Part model, mm, in its own coordinate system. A direction names the side the tool comes from. Coordinates: 2 decimals unless noted, no trailing zeros. Write each loop counter-clockwise with the first axis right and the second up, starting at its lowest first coordinate (ties: lowest second). Pieces come first, ordered by that corner, then holes. Notation, with made-up numbers: (39.25, -18.75) -> (48.25, -18.75) arc R20 cw to (48.25, -10.75) -> close; hole circle Ø7 at (44, 21). An arc over 180 degrees is marked (long way). Write item = value, one per line. Start each with the question number.
Q1. Pull direction Z, two halves, no side cores. Call faces 4 (the cylindrical face through (-31.2, 8.5, -0.1)), 5 (the flat face through (0, 3, 12.5)), 6 (the cylindrical face through (31.2, 8.7, 11.5)): released by +Z, released by -Z, zero draft, split by the parting line, or undercut.
Q2. Band-saw the part on B-B, the plane z = -0.5. List the corners of the cut face in (x, y).
Q3. Tool access for faces 1 (the cylindrical face through (31.3, 8.5, -0.1)), 2 (the flat face through (0, 3, -12.5)), 3 (the flat face through (0, 2, 10)): list every direction of +Z, -Z, +X, -X, +Y, -Y with a clear straight run to the whole face (end or side of a thin tool).
Q4. Band-saw the part on A-A, the plane x = 16.5. List the corners of the cut face in (y, z), plus the area to 3 significant figures.
Q5. Probe line 1 (Z direction, x = -24.5, y = 2.75); line 2 (X direction, y = 1.75, z = -1); line 3 (X direction, y = 5.5, z = 10.75). List the from-to ranges inside material, lowest first.
Q6. Band-saw the part on D-D, the plane y = 3. List the corners of the cut face in (x, z).
Q7. Band-saw the part on C-C, the plane y = 7. List the corners of the cut face in (x, z), plus the area to 3 significant figures.
Q8. Pin check, flat tip, straight feed: P1, Ø1.5, axis at x = 21, z = -3.5, coming from the +Y side. Stop position of the tip, or through.
Autodesk Inventor part; units mm, degrees
ref_plane "YZ Plane" through (0, 0, 0) normal (1, 0, 0) x (0, 1, 0)
ref_plane "XZ Plane" through (0, 0, 0) normal (0, 1, 0) x (-1, 0, 0)
ref_plane "XY Plane" through (0, 0, 0) normal (0, 0, 1) x (1, 0, 0)
sketch "Sketch1" plane through (0, 0, 0) normal (0, 1, 0) x (-1, 0, 0)
  line L0 (-35, -12.5) -> (35, -12.5)
  line L1 (35, -12.5) -> (35, 12.5)
  line L2 (35, 12.5) -> (-35, 12.5)
  line L3 (-35, 12.5) -> (-35, -12.5)
  line L4 (-35, -12.5) -> (35, 12.5) construction
  line L5 (35, -12.5) -> (-35, 12.5) construction
  line L6 (-24.5, -5) -> (24.5, -5) construction
  line L7 (24.5, -5) -> (24.5, 5) construction
  line L8 (24.5, 5) -> (-24.5, 5) construction
  line L9 (-24.5, 5) -> (-24.5, -5) construction
  line L10 (-24.5, -5) -> (24.5, 5) construction
  line L11 (24.5, -5) -> (-24.5, 5) construction
  circle A0 centre (24.5, 5) radius 2.25
  circle A1 centre (24.5, -5) radius 2.25
  circle A2 centre (-24.5, -5) radius 2.25
  circle A3 centre (-24.5, 5) radius 2.25
  line L12 (-20, -10) -> (20, -10)
  line L13 (20, -10) -> (20, 10)
  line L14 (20, 10) -> (-20, 10)
  line L15 (-20, 10) -> (-20, -10)
  line L16 (-20, -10) -> (20, 10) construction
  line L17 (20, -10) -> (-20, 10) construction
  point P0 (0, 0)
  dimension "d0" = 10
  dimension "d1" = 49
  dimension "d2" = 4.5
  dimension "d5" = 25
  dimension "d6" = 70
  dimension "d7" = 20
  dimension "d8" = 40
extrude "Extrusion1" add sketch "Sketch1" along normal blind 5
sketch "Sketch2" plane through (35, 0, -12.5) normal (0, 0, -1) x (-1, 0, 0)
  line L0 (62.5, 5) -> (62.5, 11)
  line L1 (62.5, 11) -> (70, 11)
  line L2 (70, 11) -> (70, 5)
  line L3 (70, 5) -> (62.5, 5)
  line L4 (35, -3.7897) -> (35, 10.3895) construction
  circle A0 centre (66.25, 11) radius 2.5
  line L5 (0, 5) -> (7.5, 5)
  circle A1 centre (66.25, 11) radius 2.3
  line L6 (7.5, 5) -> (7.5, 11)
  line L7 (7.5, 11) -> (0, 11)
  line L8 (0, 11) -> (0, 5)
  line L9 (0, 5) -> (7.5, 5)
  circle A2 centre (3.75, 11) radius 2.5
  circle A3 centre (3.75, 11) radius 2.3
  line L10 (0, 0) -> (70, 0)
  point P0 (35, 0)
  point P1 (35, 0)
  point P2 (68.75, 11)
  point P3 (63.75, 11)
  point P4 (35, 0)
  point P5 (6.05, 11)
  point P6 (1.45, 11)
  point P7 (1.25, 11)
  point P8 (6.25, 11)
  point P9 (68.55, 11)
  point P10 (63.95, 11)
  dimension "d9" = 5
  dimension "d10" = 7.5
  dimension "d12" = 6
  dimension "d18" = 0.2
extrude "Extrusion2" add sketch "Sketch2" against normal up to surface (25 mm away) contours L0 L1 A0 L2 L3 | L8 L7 A2 L6 L5
extrude "Extrusion4" add sketch "Sketch2" against normal blind 2 contours L1 A1 A0 | L7 A3 A2 picked at (64.2095, 9.7038) picked at (6.1368, 10.6171)
mirror "Mirror1" about plane through (0, 0, 0) normal (0, 0, 1) of "Extrusion4"
properties part number "Servo mount"
Ans:
q1.face_4 = undercut
q1.face_5 = released by +Z
q1.face_6 = zero draft
q2.outline = (-35, 0) -> (-20, 0) -> (-20, 5) -> (-27.5, 5) -> (-27.5, 11) -> (-28.75, 11) arc R2.5 cw to (-33.75, 11) -> (-35, 11) -> close; (20, 0) -> (35, 0) -> (35, 11) -> (33.75, 11) arc R2.5 cw to (28.75, 11) -> (27.5, 11) -> (27.5, 5) -> (20, 5) -> close
q3.face_1 = +Y
q3.face_2 = -Z, +X, -X, +Y, -Y
q3.face_3 = +Y, -Y
q4.outline = (0, -12.5) -> (5, -12.5) -> (5, -10) -> (0, -10) -> close; (0, 10) -> (5, 10) -> (5, 12.5) -> (0, 12.5) -> close
q4.area = 25.0 mm2
q5.line_1 = -12.5 to -7.25, -2.75 to 2.75, 7.25 to 12.5
q5.line_2 = -35 to -20, 20 to 35
q5.line_3 = -35 to -27.5, 27.5 to 35
q6.outline = (-35, -12.5) -> (35, -12.5) -> (35, 12.5) -> (-35, 12.5) -> close; hole circle Ø4.5 at (-24.5, -5); hole circle Ø4.5 at (-24.5, 5); hole (-20, -10) -> (20, -10) -> (20, 10) -> (-20, 10) -> close; hole circle Ø4.5 at (24.5, -5); hole circle Ø4.5 at (24.5, 5)
q7.outline = (-35, -12.5) -> (-27.5, -12.5) -> (-27.5, 12.5) -> (-35, 12.5) -> close; (27.5, -12.5) -> (35, -12.5) -> (35, 12.5) -> (27.5, 12.5) -> close
q7.area = 375 mm2
q8.P1 = 5
